Could you check a few things on this model? Use its own coordinates, in mm. Round coordinates to 2 decimals unless told otherwise and drop trailing zeros. Write each loop counter-clockwise with the first axis right and the second up, starting at its lowest first coordinate (ties: lowest second). Pieces come first, ordered by that corner, then holes. Notation, with made-up numbers: M 36,6.5 L 94,6.5 A18 ccw 94,25.5 Z; hole C -13.75,88.5 d10. An arc over 180 degrees is marked long. One line per item, written item: value. Start each with the question number.
(1) I'm going to push flat-ended pins straight in: pin 1 Ø1 at (y, z) = (-11, -12) entering from +X; pin 2 Ø4 at (y, z) = (14.5, -15.5) entering from -X; pin 3 Ø10 at (x, y) = (-15.5, -1.5) entering from -Z. Where does each tip first touch, or does it pass through?
(2) I want a section at A-A on x = 17. Please give me the cut outline in (y, z).
(3) I want a section at C-C on x = -11.5. Please give me the cut outline in (y, z).
(4) I want a section at B-B on z = 8. Please give me the cut outline in (x, y).
(5) If I drill on L1, parallel to X at y = 17.5, z = -8; L2, parallel to X at y = 1, z = -6; L3, parallel to Y at x = -4, z = -1.5, over which ranges is the centre line in solid material (lowest first)?
```python
from build123d import *

# Parameters (mm, degrees)
F0_W     = 38.1
F0_H     = 40.64
F1_DEPTH = 50.8
F3_DEPTH = 25.4
F4_R     = 7.62
F5_R     = 2.54
F6_R     = 2.54
F7_R     = 5.08


with BuildPart() as f1:
    # F0 (on Right) → F1 (new body)
    with BuildSketch(Plane.YZ):
        with Locations((3.9571700618, -0.6121383074)):
            Rectangle(F0_W, F0_H)
    extrude(amount=F1_DEPTH)

    # F2 (on face) → F3 (join)
    with BuildSketch(Plane(origin=(0, 0, 0), x_dir=(0, -1, 0), z_dir=(-1, 0, 0))):
        with BuildLine():
            Line((-3.9571700618, -6.9621383074), (-3.9571700618, -0.6121383074))
            Line((-3.9571700618, -0.6121383074), (-10.3071700618, -0.6121383074))
            ThreePointArc((-10.3071700618, -0.6121383074), (-8.4472981223, -5.1022663679), (-3.9571700618, -6.9621383074))
        make_face()
        with BuildLine():
            ThreePointArc((-3.9571700618, -6.9621383074), (0.5329579988, -5.1022663679), (2.3928299382, -0.6121383074))
            Line((2.3928299382, -0.6121383074), (-3.9571700618, -0.6121383074))
            Line((-3.9571700618, -0.6121383074), (-3.9571700618, -6.9621383074))
        make_face()
        with BuildLine():
            Line((-10.3071700618, -0.6121383074), (-3.9571700618, -0.6121383074))
            Line((-3.9571700618, -0.6121383074), (-3.9571700618, 5.7378616926))
            ThreePointArc((-3.9571700618, 5.7378616926), (-8.4472981223, 3.8779897531), (-10.3071700618, -0.6121383074))
        make_face()
        with BuildLine():
            Line((-3.9571700618, -0.6121383074), (2.3928299382, -0.6121383074))
            ThreePointArc((2.3928299382, -0.6121383074), (0.5329579988, 3.8779897531), (-3.9571700618, 5.7378616926))
            Line((-3.9571700618, 5.7378616926), (-3.9571700618, -0.6121383074))
        make_face()
    extrude(amount=F3_DEPTH)

    # F4
    f4_edges = [f1.edges().sort_by_distance(p)[0] for p in [
        (25.4, 23.00717, -20.932138),
        (25.4, -15.09283, -20.932138),
        (25.4, -15.09283, 19.707862),
        (25.4, 23.00717, 19.707862),
    ]]
    fillet(f4_edges, radius=F4_R)

    # F5
    f5_edges = [f1.edges().sort_by_distance(p)[0] for p in [
        (0, 3.95717, -20.932138),
    ]]
    fillet(f5_edges, radius=F5_R)

    # F6
    f6_edges = [f1.edges().sort_by_distance(p)[0] for p in [
        (-25.4, 10.30717, -0.612138),
    ]]
    fillet(f6_edges, radius=F6_R)

    # F7
    f7_edges = [f1.edges().sort_by_distance(p)[0] for p in [
        (50.8, 3.95717, 19.707862),
        (50.8, -12.860984, 17.476015),
        (50.8, -15.09283, -0.612138),
        (50.8, -12.860984, -18.700292),
        (50.8, 3.95717, -20.932138),
        (50.8, 23.00717, -0.612138),
        (50.8, 20.775324, 17.476015),
        (50.8, 20.775324, -18.700292),
    ]]
    fillet(f7_edges, radius=F7_R)


solid = f1.part
```
Found:
1. pin 1: stops at x = 50.78
1. pin 2: stops at x = 0
1. pin 3: stops at z = -6.95
2. outline: M -15.09,-13.31 A7.62 ccw -7.47,-20.93 L 15.39,-20.93 A7.62 ccw 23.01,-13.31 L 23.01,12.09 A7.62 ccw 15.39,19.71 L -7.47,19.71 A7.62 ccw -15.09,12.09 Z
3. outline: C 3.96,-0.61 d12.7
4. outline: M 0,-12.55 A2.54 ccw 2.54,-15.09 L 45.72,-15.09 A5.08 ccw 50.8,-10.01 L 50.8,17.93 A5.08 ccw 45.72,23.01 L 2.54,23.01 A2.54 ccw 0,20.47 Z
5. L1: x = 0 to 50.8
5. L2: x = -23.86 to 50.8
5. L3: y = -2.33 to 10.24
